Build history of the part. All positions in model axes, mm. A direction names the side the tool comes from. Give positions to 0.01 mm unless a question says otherwise; leave off trailing zeros. Loops run counter-clockwise (first coordinate to the right, second up) from the corner with the lowest first, then second, coordinate; pieces in that order, holes last.
1) Flat gauge pins, fed straight in: P1, Ø10, axis at x = -40, y = 63, coming from the -Z side; P2, Ø6, axis at y = 68.5, z = 47.5, coming from the -X side; P3, Ø1.5, axis at y = 3.5, z = -24, coming from the +X side. Where does each tip first touch, or does it go through?
2) Band-saw the part on A-A on x = -10. List the corners of the cut face in (y, z).
3) Wall check: line 1 (X direction, y = 64.5, z = 36.5); line 2 (Z direction, x = -26, y = 37.5); line 3 (Y direction, x = -48.5, z = 40.5). Give the ranges that are in metal, low to high.
4) Band-saw the part on B-B on z = -2. List the corners of the cut face in (x, y), then the cut area to 3 significant figures.
5) Band-saw the part on D-D on z = -17. List the corners of the cut face in (x, y), then the cut area to 3 significant figures.
6) Two-plate mould, pull along X, no slides. Class faces 4 (the flat face through (42, 2, -21)), 5 (the cylindrical face through (-73.818, 2.535, 0.059)), 6 (the cylindrical face through (36.96, 2.54, -63.9)), 7 (the flat face through (36, 85, 0)): +X half, -X half, draft (parallel to the pull), parting line (faces both ways), or undercut.
7) 3-axis set-ups, long thin cutter, end or side, ignore diameter. For faces 1 (the flat face through (40, 44, -1)), 2 (the cylindrical face through (37.594, 44.44, -62.719)), 3 (the cylindrical face through (-37.594, 44.44, 62.719)): which of +Z, -Z, +X, -X, +Y, -Y reach the whole face in a straight line?
8) Band-saw the part on C-C on y = 57. List the corners of the cut face in (x, z), then the cut area to 3 significant figures.
```python
from build123d import *

# Parameters (mm, degrees)
BOSS_EXTRUDE1_DEPTH = 5
FILLET1_R           = 8
BOSS_EXTRUDE2_DEPTH = 80
CUT_EXTRUDE1_DEPTH  = 85
CUT_EXTRUDE2_DEPTH  = 5


with BuildPart() as part:
    # Sketch1 → Boss-Extrude1 (new body)
    with BuildSketch(Plane(origin=(0, 0, 0), x_dir=(1, 0, 0), z_dir=(0, 1, 0))):
        Polygon((-75.055534995, 0), (-37.527767497, -65), (37.527767497, -65), (75.055534995, 0), (37.527767497, 65), (-37.527767497, 65), align=None)
    extrude(amount=BOSS_EXTRUDE1_DEPTH)

    # Fillet1
    fillet1_edges = [part.edges().sort_by_distance(p)[0] for p in [
        (-37.527767497, 2.5, -65),
        (37.527767497, 2.5, -65),
        (75.055534995, 2.5, 0),
        (37.527767497, 2.5, 65),
        (-37.527767497, 2.5, 65),
        (-75.055534995, 2.5, 0),
    ]]
    fillet(fillet1_edges, radius=FILLET1_R)

    # Sketch3 → Boss-Extrude2 (add)
    with BuildSketch(Plane(origin=(0, 5, 0), x_dir=(1, 0, 0), z_dir=(0, 1, 0))):
        with BuildLine():
            Line((-32, 65), (32, 65))
            ThreePointArc((32, 65), (37.656854249, 62.656854249), (40, 57))
            Line((40, 57), (40, -57))
            ThreePointArc((40, -57), (37.656854249, -62.656854249), (32, -65))
            Line((32, -65), (-32, -65))
            ThreePointArc((-32, -65), (-37.656854249, -62.656854249), (-40, -57))
            Line((-40, -57), (-40, 57))
            ThreePointArc((-40, 57), (-37.656854249, 62.656854249), (-32, 65))
        make_face()
    extrude(amount=BOSS_EXTRUDE2_DEPTH)

    # Sketch4 → Cut-Extrude1 (cut)
    with BuildSketch(Plane(origin=(0, 85, 0), x_dir=(1, 0, 0), z_dir=(0, 1, 0))):
        Polygon((-35, 57), (-32, 60), (32, 60), (35, 57), (35, -57), (32, -60), (-32, -60), (-35, -57), align=None)
    extrude(amount=-CUT_EXTRUDE1_DEPTH, mode=Mode.SUBTRACT)

    # Sketch8 → Cut-Extrude2 (cut)
    with BuildSketch(Plane(origin=(0, 0, 0), x_dir=(1, 0, 0), z_dir=(0, 1, 0))):
        with BuildLine():
            ThreePointArc((58.889727457, 8), (58.889727457, 6), (57.15767665, 5))
            Line((57.15767665, 5), (42, 5))
            Line((42, 5), (42, 37.253866082))
            Line((42, 37.253866082), (58.889727457, 8))
        make_face()
        with BuildLine():
            Line((42, -37.253866082), (58.889727457, -8))
            ThreePointArc((58.889727457, -8), (58.889727457, -6), (57.15767665, -5))
            Line((57.15767665, -5), (42, -5))
            Line((42, -5), (42, -37.253866082))
        make_face()
        with BuildLine():
            ThreePointArc((-58.889727457, -8), (-58.889727457, -6), (-57.15767665, -5))
            Line((-57.15767665, -5), (-42, -5))
            Line((-42, -5), (-42, -37.253866082))
            Line((-42, -37.253866082), (-58.889727457, -8))
        make_face()
        with BuildLine():
            Line((-42, 37.253866082), (-58.889727457, 8))
            ThreePointArc((-58.889727457, 8), (-58.889727457, 6), (-57.15767665, 5))
            Line((-57.15767665, 5), (-42, 5))
            Line((-42, 5), (-42, 37.253866082))
        make_face()
    extrude(amount=CUT_EXTRUDE2_DEPTH, mode=Mode.SUBTRACT)


solid = part.part
```
Findings below:
1. P1: stops at z = -64.42
1. P2: stops at x = -40
1. P3: stops at x = 61.63
2. outline: (0, -65) - (85, -65) - (85, -60) - (0, -60) - close; (0, 60) - (85, 60) - (85, 65) - (0, 65) - close
3. line 1: x = -40 to -35, 35 to 40
3. line 2: z = -65 to -60, 60 to 65
3. line 3: y = 0 to 5
4. outline: (-73.56, 0) - (-35, 0) - (-35, 85) - (-40, 85) - (-40, 5) - (-73.56, 5) - close; (35, 0) - (73.56, 0) - (73.56, 5) - (40, 5) - (40, 85) - (35, 85) - close
4. area: 1,190 mm2
5. outline: (-65.24, 0) - (-53.69, 0) - (-53.69, 5) - (-65.24, 5) - close; (-42, 0) - (-35, 0) - (-35, 85) - (-40, 85) - (-40, 5) - (-42, 5) - close; (35, 0) - (42, 0) - (42, 5) - (40, 5) - (40, 85) - (35, 85) - close; (53.69, 0) - (65.24, 0) - (65.24, 5) - (53.69, 5) - close
5. area: 985 mm2
6. face 4: undercut
6. face 5: -X half
6. face 6: +X half
6. face 7: draft
7. face 1: +Z, -Z, +X, +Y
7. face 2: -Z, +X, +Y
7. face 3: +Z, -X, +Y
8. outline: (-40, -57) arc R8 ccw to (-32, -65) - (32, -65) arc R8 ccw to (40, -57) - (40, 57) arc R8 ccw to (32, 65) - (-32, 65) arc R8 ccw to (-40, 57) - close; hole (-35, -57) - (-32, -60) - (32, -60) - (35, -57) - (35, 57) - (32, 60) - (-32, 60) - (-35, 57) - close
8. area: 1,960 mm2
